The listing builds one solid part. Answer for the finished solid, in the listing's coordinates (mm). A direction names the side the tool comes from. Give positions to 0.01 mm unless a question says otherwise; leave off trailing zeros. Loops run counter-clockwise (first coordinate to the right, second up) from the corner with the lowest first, then second, coordinate; pieces in that order, holes last. Notation, with made-up numbers: M 33.25,23 L 54.25,23 A20 ccw 54.25,61 Z; hole C -11.5,-27 d8. An arc over 180 degrees is marked long. One line per item, written item: value. Start each with the question number.
Q1. For faces 5 (the cylindrical face through (-1.43, 10.9, 14.01)), 6 (the flat face through (-3, 5, 2)), determine the directions among +Z, -Z, +X, -X, +Y, -Y from which every point of the face is accessible in a straight line to the end or side of a thin tool.
Q2. A cutting plane is placed at D-D, the plane x = 4.25. Determine the outline of the cut face in (y, z).
Q3. A cutting plane is placed at C-C, the plane z = 3.25. Determine the outline of the cut face in (x, y), and give its area (3 significant figures).
Q4. A cutting plane is placed at A-A, the plane y = 0. Determine the outline of the cut face in (x, z).
Q5. The mould has two halves that part along Z. Classify faces 1 (the flat face through (-3, 5, 13)), 2 (the flat face through (0, -2, 0)), 3 (the flat face through (0, -2, 15)), 4 (the cylindrical face through (-1.43, 10.9, 0.99)): +Z half, -Z half, draft (parallel to the pull), parting line (faces both ways), or undercut.
Q6. Consider L1, parallel to Z at x = -5.25, y = 7.25; L2, parallel to Y at x = 1, z = 5.75; L3, parallel to X at y = 2, z = 14.25. Determine where each line is inside the solid, lowest interval first.
Q7. Flat-ended cylindrical pins translate along their axes: pin 1 (0.6 mm diameter, centred on x = -0.5, z = 14.5, fed in from +Y); pin 2 (3 mm diameter, centred on x = -6, z = 7, fed in from -Y); pin 3 (2.5 mm diameter, centred on y = 0, z = 11, fed in from +X). Find the tip coordinate at first contact, or state that the pin passes through.
from build123d import *

# Parameters (mm, degrees)
SKETCH_1_R      = 10.992648621
SKETCH_1_W      = 3
SKETCH_1_H      = 3
EXTRUDE_1_DEPTH = 2
SKETCH_2_R      = 5.5
SKETCH_2_W      = 3
SKETCH_2_H      = 3
EXTRUDE_2_DEPTH = 5.5


with BuildPart() as part:
    # 草图1 → 凸台-拉伸1 (new body)
    with BuildSketch(Plane.XY):
        Circle(SKETCH_1_R)
        Rectangle(SKETCH_1_W, SKETCH_1_H, mode=Mode.SUBTRACT)
    extrude_1 = extrude(amount=EXTRUDE_1_DEPTH)

    # 草图2 → 凸台-拉伸2 (add)
    with BuildSketch(Plane.XY.offset(2)):
        Circle(SKETCH_2_R)
        Rectangle(SKETCH_2_W, SKETCH_2_H, mode=Mode.SUBTRACT)
    extrude_2 = extrude(amount=EXTRUDE_2_DEPTH)

    # 镜向1: 凸台-拉伸1, 凸台-拉伸2 across plane
    add(extrude_1.mirror(Plane.XY.offset(7.5)))
    add(extrude_2.mirror(Plane.XY.offset(7.5)))


solid = part.part
Answer block:
1. face 5: +Z, -Z
1. face 6: none
2. outline: M -10.14,0 L 10.14,0 L 10.14,2 L 3.49,2 L 3.49,13 L 10.14,13 L 10.14,15 L -10.14,15 L -10.14,13 L -3.49,13 L -3.49,2 L -10.14,2 Z
3. outline: C 0,0 d11; hole M -1.5,-1.5 L 1.5,-1.5 L 1.5,1.5 L -1.5,1.5 Z
3. area: 86.0 mm^2
4. outline: M -10.99,0 L -1.5,0 L -1.5,15 L -10.99,15 L -10.99,13 L -5.5,13 L -5.5,2 L -10.99,2 Z; M 1.5,0 L 10.99,0 L 10.99,2 L 5.5,2 L 5.5,13 L 10.99,13 L 10.99,15 L 1.5,15 Z
5. face 1: undercut
5. face 2: -Z half
5. face 3: +Z half
5. face 4: draft
6. L1: 0 to 2, 13 to 15
6. L2: -5.41 to -1.5, 1.5 to 5.41
6. L3: -10.81 to 10.81
7. pin 1: y = 10.99
7. pin 2: y = -3.16
7. pin 3: x = 5.5
